Design review of the part built by this model. Coordinates are the model's own, in mm. A direction names the side the tool comes from. Coordinates: 2 decimals unless noted, no trailing zeros. Write each loop counter-clockwise with the first axis right and the second up, starting at its lowest first coordinate (ties: lowest second). Pieces come first, ordered by that corner, then holes. Notation, with made-up numbers: M 2,79.25 L 32,79.25 A37 ccw 32,118.25 Z; hole C 6.5,24 d7. An arc over 180 degrees is marked long. Return JSON: item names as keys, results as strings. Group by question number.
```python
from build123d import *

# Parameters (mm, degrees)
SKETCH_1_W             = 24
SKETCH_1_H             = 3
EXTRUDE_1_DEPTH        = 88
FILLET_1_R             = 2
SKETCH_3_R             = 2.05
CUT_EXTRUDE_1_DEPTH    = 89.865066252
SKETCH_4_R             = 4
CUT_EXTRUDE_2_DEPTH    = 89.865066252
PATTERN_LINEAR_1_COUNT = 12
PATTERN_LINEAR_1_PITCH = 16
PATTERN_LINEAR_2_COUNT = 11
PATTERN_LINEAR_2_PITCH = 16
SKETCH_5_R             = 2.05
CUT_EXTRUDE_3_DEPTH    = 89.865066252
SKETCH_6_W             = 4.2
SKETCH_6_H             = 3
CUT_EXTRUDE_4_DEPTH    = 66
SKETCH_7_R             = 2.05
CUT_EXTRUDE_5_DEPTH    = 10


with BuildPart() as part:
    # 草图1 → 凸台-拉伸1 (new body)
    with BuildSketch(Plane(origin=(0, 0, 0), x_dir=(0, 0, -1), z_dir=(1, 0, 0))):
        Rectangle(SKETCH_1_W, SKETCH_1_H)
    extrude(amount=EXTRUDE_1_DEPTH)

    # 圆角1
    fillet_1_edges = [part.edges().sort_by_distance(p)[0] for p in [
        (88, 0, 12),
        (88, 0, -12),
        (0, 0, 12),
        (0, 0, -12),
    ]]
    fillet(fillet_1_edges, radius=FILLET_1_R)

    # 草图3 → 切除-拉伸1 (cut, through all)
    with BuildSketch(Plane(origin=(0, 1.5, 0), x_dir=(1, 0, 0), z_dir=(0, 1, 0))):
        with Locations(Location((4, 8, 0), (0, 0, 270))):
            Circle(SKETCH_3_R)
        with Locations(Location((4, -8, 0), (0, 0, 270))):
            Circle(SKETCH_3_R)
    cut_extrude_1 = extrude(amount=-CUT_EXTRUDE_1_DEPTH, mode=Mode.SUBTRACT)

    # 草图4 → 切除-拉伸2 (cut, through all)
    with BuildSketch(Plane(origin=(0, 1.5, 0), x_dir=(1, 0, 0), z_dir=(0, 1, 0))):
        with Locations(Location((12, 0, 0), (0, 0, 270))):
            Circle(SKETCH_4_R)
    cut_extrude_2 = extrude(amount=-CUT_EXTRUDE_2_DEPTH, mode=Mode.SUBTRACT)

    # 阵列(线性)1: 切除-拉伸1 ×12
    with Locations(*[(i * PATTERN_LINEAR_1_PITCH, 0, 0) for i in range(1, PATTERN_LINEAR_1_COUNT)]):
        add(cut_extrude_1, mode=Mode.SUBTRACT)

    # 阵列(线性)2: 切除-拉伸2 ×11
    with Locations(*[(i * PATTERN_LINEAR_2_PITCH, 0, 0) for i in range(1, PATTERN_LINEAR_2_COUNT)]):
        add(cut_extrude_2, mode=Mode.SUBTRACT)

    # 草图5 → 切除-拉伸3 (cut, through all)
    with BuildSketch(Plane(origin=(0, 1.5, 0), x_dir=(1, 0, 0), z_dir=(0, 1, 0))):
        with Locations(Location((4, 0, 0), (0, 0, 270))):
            Circle(SKETCH_5_R)
        with Locations(Location((84, 0, 0), (0, 0, 270))):
            Circle(SKETCH_5_R)
    extrude(amount=-CUT_EXTRUDE_3_DEPTH, mode=Mode.SUBTRACT)

    # 草图6 → 切除-拉伸4 (cut)
    with BuildSketch(Plane.ZY.offset(-12)):
        Rectangle(SKETCH_6_W, SKETCH_6_H)
    extrude(amount=-CUT_EXTRUDE_4_DEPTH, mode=Mode.SUBTRACT)

    # 草图7 → 切除-拉伸5 (cut)
    with BuildSketch(Plane(origin=(0, 1.5, 0), x_dir=(1, 0, 0), z_dir=(0, 1, 0))):
        with Locations(Location((12, 8, 0), (0, 0, 270))):
            Circle(SKETCH_7_R)
        with Locations(Location((12, -8, 0), (0, 0, 270))):
            Circle(SKETCH_7_R)
    cut_extrude_5 = extrude(amount=-CUT_EXTRUDE_5_DEPTH, mode=Mode.SUBTRACT)

    # 镜向1: 切除-拉伸5 across plane
    add(cut_extrude_5.mirror(Plane.ZY.offset(-44)), mode=Mode.SUBTRACT)


solid = part.part
```
Item 1: Machinability: for faces 1 (the flat face through (36, 0, 2.1)), 2 (the flat face through (43, 0, -12)), which of the approach directions +Z, -Z, +X, -X, +Y, -Y give a long, thin tool a straight path to every point of the face, cutting with its end or side? Answer none if there is none.
Item 2: For line 1 (X direction, y = 0.4, z = 0); line 2 (X direction, y = 1.2, z = -1); line 3 (Z direction, x = 56, y = 0.05), list the stretches that pass through material, from the lowest coordinate up.
Item 3: Add section B-B (y = 0.55). Count the separate pieces of the cut face and the enclosed holes in it, plus the area to 3 significant figures.
Item 4: The part is to be moulded in two halves that separate along X. For faces 3 (the cylindrical face through (0.6, 0.02, -11.43)), 4 (the flat face through (36, 0, -2.1)), 5 (the flat face through (43, 0, 12)), say which applies: pulls with the +X half, pulls with the -X half, needs draft (parallel to the pull), parting line crosses it, or undercut.
Item 5: For pin 1 (6.5 mm diameter, centred on x = 4, z = 8, fed in from -Y); pin 2 (3.5 mm diameter, centred on x = 12, z = -8, fed in from +Y), all flat-tipped, find the tip position at first contact; note any pin that passes through.
Item 6: Add section A-A (x = 52). Write out the cut boundary in (y, z), plus the area to 3 significant figures.
Geometry check:
{
 "1": {"face 1": "+Y, -Y", "face 2": "-Z, +X, -X, +Y, -Y"},
 "2": {"line 1": "0 to 1.95, 6.05 to 8, 80 to 81.95, 86.05 to 88", "line 2": "0 to 2.21, 5.79 to 8.13, 79.87 to 82.21, 85.79 to 88", "line 3": "-12 to -2.1, 2.1 to 12"},
 "3": {"separate pieces": "1", "enclosed holes": "19", "area": "1,480 mm^2"},
 "4": {"face 3": "pulls with the -X half", "face 4": "undercut", "face 5": "needs draft"},
 "5": {"pin 1": "y = -1.5", "pin 2": "through"},
 "6": {"outline": "M -1.5,-12 L 1.5,-12 L 1.5,-10.05 L -1.5,-10.05 Z; M -1.5,-5.95 L 1.5,-5.95 L 1.5,-2.1 L -1.5,-2.1 Z; M -1.5,2.1 L 1.5,2.1 L 1.5,5.95 L -1.5,5.95 Z; M -1.5,10.05 L 1.5,10.05 L 1.5,12 L -1.5,12 Z", "area": "34.8 mm^2"}
}
